```python
from build123d import *

# Parameters (mm, degrees)
ESQUISSE2_W      = 18
ESQUISSE2_H      = 18
EXTRUSION1_DEPTH = 15


with BuildPart() as part:
    # Esquisse1 → Révolution1 (revolve)
    with BuildSketch(Plane.XY):
        with BuildLine():
            Line((-12, 36.538644398), (-12, 34))
            Line((-12, 34), (-8, 34))
            Line((-8, 34), (-8, 29))
            Line((-8, 29), (-10, 29))
            Line((-10, 29), (-10, 20))
            Line((-10, 20), (-8, 20))
            Line((-8, 20), (-8, 0))
            Line((-8, 0), (0, 0))
            Line((0, 0), (0, 38))
            ThreePointArc((0, 38), (-6.044327096, 37.633316532), (-12, 36.538644398))
        make_face()
    revolve(axis=Axis((0, 0, 0), (0, 1, 0)))

    # Esquisse2 → Extrusion1 (add)
    with BuildSketch(Plane.XZ):
        Rectangle(ESQUISSE2_W, ESQUISSE2_H)
    extrude(amount=EXTRUSION1_DEPTH)


solid = part.part
```
The listing builds one solid part. Answer for the finished solid, in the listing's coordinates (mm). A direction names the side the tool comes from. Round coordinates to 2 decimals unless told otherwise and drop trailing zeros. Loops run counter-clockwise (first coordinate to the right, second up) from the corner with the lowest first, then second, coordinate; pieces in that order, holes last.
Q1. Section A-A, the plane x = 0 is taken. Determine the outline of the cut face in (y, z).
Q2. Find the intervals of material crossed by line 1 (Y direction, x = -0.25, z = 8.75); line 2 (Y direction, x = -3.75, z = -7.5); line 3 (Z direction, x = 4.25, y = -1), in increasing order.
Q3. Section B-B, the plane z = 0 is taken. Determine the outline of the cut face in (x, y).
Q4. Given pin 1 Ø7.5 at (x, y) = (1.5, -11) entering from -Z; pin 2 Ø8 at (x, y) = (1, 28) entering from +Z; pin 3 Ø1.5 at (x, z) = (6, 1.5) entering from +Y, each flat-ended and moving along its own axis, determine where each tip first touches the part or whether it passes through.
Q5. For a pull along Y with two mould halves and no side action, classify faces 1 (the face through (0, -15, 0)), 2 (the face through (1.73, 31.46, -7.81)), 3 (the face through (2.17, 24.44, -9.76)), 4 (the face through (9, -7, 0)) as released by +Y, released by -Y, zero draft, split by the parting line, or undercut.
Q6. Section D-D, the plane y = 11 is taken. Determine the outline of the cut face in (x, z), then the cut area to 3 significant figures.
Q7. Section C-C, the plane y = -7 is taken. Determine the outline of the cut face in (x, z), then the cut area to 3 significant figures.
Q8. Which of the six approach directions +Z, -Z, +X, -X, +Y, -Y give full straight-line access (tool end or side, diameter ignored) to faces 5 (the face through (0, -7, 9)), 6 (the face through (0, 20, 8.2)), 7 (the face through (-9, -7, 0))?
Completed:
1. outline: (-15, -9) - (0, -9) - (0, -8) - (20, -8) - (20, -10) - (29, -10) - (29, -8) - (34, -8) - (34, -12) - (36.54, -12) arc R50 ccw to (36.54, 12) - (34, 12) - (34, 8) - (29, 8) - (29, 10) - (20, 10) - (20, 8) - (0, 8) - (0, 9) - (-15, 9) - close
2. line 1: y = -15 to 0, 20 to 29, 34 to 37.23
2. line 2: y = -15 to 0, 20 to 29, 34 to 37.29
2. line 3: z = -9 to 9
3. outline: (-12, 34) - (-8, 34) - (-8, 29) - (-10, 29) - (-10, 20) - (-8, 20) - (-8, 0) - (-9, 0) - (-9, -15) - (9, -15) - (9, 0) - (8, 0) - (8, 20) - (10, 20) - (10, 29) - (8, 29) - (8, 34) - (12, 34) - (12, 36.54) arc R50 ccw to (-12, 36.54) - close
4. pin 1: stops at z = -9
4. pin 2: stops at z = 10
4. pin 3: stops at y = 37.7
5. face 1: released by -Y
5. face 2: undercut
5. face 3: undercut
5. face 4: zero draft
6. outline: circle Ø16 at (0, 0)
6. area: 201 mm2
7. outline: (-9, -9) - (9, -9) - (9, 9) - (-9, 9) - close
7. area: 324 mm2
8. face 5: +Z, +X, -X, -Y
8. face 6: none
8. face 7: +Z, -Z, -X, -Y
